Verification items for the finished model (mm, model axes). Give positions to 0.01 mm unless a question says otherwise; leave off trailing zeros. Order: outer loops, then holes, each group sorted by start corner. A loop starts at its lowest first (then second) coordinate and runs counter-clockwise, first axis right, second up. Notation, with made-up numbers: (-24, -26.5) - (18, -26.5) arc R13 ccw to (18, -17.5) - close; hole circle Ø11 at (15.25, -17.75). An arc over 180 degrees is marked (long way). Answer as a JSON object with one key per item and string values. Group by question number.
(1) Thickness scan on line 1 (X direction, y = 3, z = 0.8); line 2 (Y direction, x = -50.5, z = 0.75); line 3 (X direction, y = -9.5, z = 0.15). Record the ranges inside material, lowest first.
(2) Section check A-A (z = 0.65). Count the separate pieces of the cut face and the enclosed holes in it, then the cut area to 3 significant figures.
(3) Depth check by flat-ended pin: pin 1 Ø0.5 at (x, z) = (-232.5, 0.5) entering from -Y; pin 2 Ø0.5 at (x, z) = (232.5, 0.5) entering from +Y; pin 3 Ø0.5 at (y, z) = (21, 0.5) entering from -X. Enter the tip coordinate at first touch or a pass-through.
(4) Section check B-B (y = 28). Record the boundary of the cut face in (x, z).
```python
from build123d import *

# Parameters (mm, degrees)
F1_DEPTH = 1
F3_D     = 5
F5_DEPTH = 25
F7_DEPTH = 25


with BuildPart() as f1:
    # F0 (on Top) → F1 (new body)
    with BuildSketch(Plane.XY):
        Polygon((221, 20), (221, 33.5), (0, 33.5), (-221, 33.5), (-221, 20), (-223, 20), (-223, 22), (-239, 22), (-241, 20), (-241, 0), (-241, -20), (-239, -22), (-223, -22), (-223, -20), (-221, -20), (-221, -33.5), (0, -33.5), (221, -33.5), (221, -20), (223, -20), (223, -22), (239, -22), (241, -20), (241, 0), (241, 20), (239, 22), (223, 22), (223, 20), align=None)
    extrude(amount=F1_DEPTH)

    # F3 (through all)
    with Locations(Plane.XY.offset(1)):
        with Locations((-200, 0), (-100, 0), (0, 0), (100, 0), (200, 0)):
            Hole(F3_D / 2)

    # F4 (on face) → F5 (cut)
    with BuildSketch(Plane.XY.offset(1)):
        with BuildLine():
            Line((-228.9, -13), (-235, -13))
            ThreePointArc((-235, -13), (-238, -16), (-235, -19))
            Line((-235, -19), (-228.9, -19))
            ThreePointArc((-228.9, -19), (-225.9, -16), (-228.9, -13))
        make_face()
        with BuildLine():
            ThreePointArc((-235, 19), (-238, 16), (-235, 13))
            Line((-235, 13), (-228.9, 13))
            ThreePointArc((-228.9, 13), (-225.9, 16), (-228.9, 19))
            Line((-228.9, 19), (-235, 19))
        make_face()
        with BuildLine():
            Line((228.9, 13), (235, 13))
            ThreePointArc((235, 13), (238, 16), (235, 19))
            Line((235, 19), (228.9, 19))
            ThreePointArc((228.9, 19), (225.9, 16), (228.9, 13))
        make_face()
        with BuildLine():
            ThreePointArc((228.9, -13), (225.9, -16), (228.9, -19))
            Line((228.9, -19), (235, -19))
            ThreePointArc((235, -19), (238, -16), (235, -13))
            Line((235, -13), (228.9, -13))
        make_face()
    extrude(amount=-F5_DEPTH, mode=Mode.SUBTRACT)

    # F6 (on face) → F7 (cut)
    with BuildSketch(Plane(origin=(0, 0, 0), x_dir=(1, 0, 0), z_dir=(0, 0, -1))):
        with BuildLine():
            ThreePointArc((120, 12), (116.464466, 10.535534), (115, 7))
            Line((115, 7), (115, -7))
            ThreePointArc((115, -7), (116.464466, -10.535534), (120, -12))
            Line((120, -12), (180, -12))
            ThreePointArc((180, -12), (183.535534, -10.535534), (185, -7))
            Line((185, -7), (185, 7))
            ThreePointArc((185, 7), (183.535534, 10.535534), (180, 12))
            Line((180, 12), (120, 12))
        make_face()
        with BuildLine():
            ThreePointArc((20, 12), (16.464466, 10.535534), (15, 7))
            Line((15, 7), (15, -7))
            ThreePointArc((15, -7), (16.464466, -10.535534), (20, -12))
            Line((20, -12), (80, -12))
            ThreePointArc((80, -12), (83.535534, -10.535534), (85, -7))
            Line((85, -7), (85, 7))
            ThreePointArc((85, 7), (83.535534, 10.535534), (80, 12))
            Line((80, 12), (20, 12))
        make_face()
        with BuildLine():
            ThreePointArc((-15, 7), (-16.464466, 10.535534), (-20, 12))
            Line((-20, 12), (-80, 12))
            ThreePointArc((-80, 12), (-83.535534, 10.535534), (-85, 7))
            Line((-85, 7), (-85, -7))
            ThreePointArc((-85, -7), (-83.535534, -10.535534), (-80, -12))
            Line((-80, -12), (-20, -12))
            ThreePointArc((-20, -12), (-16.464466, -10.535534), (-15, -7))
            Line((-15, -7), (-15, 7))
        make_face()
        with BuildLine():
            ThreePointArc((-115, 7), (-116.464466, 10.535534), (-120, 12))
            Line((-120, 12), (-180, 12))
            ThreePointArc((-180, 12), (-183.535534, 10.535534), (-185, 7))
            Line((-185, 7), (-185, -7))
            ThreePointArc((-185, -7), (-183.535534, -10.535534), (-180, -12))
            Line((-180, -12), (-120, -12))
            ThreePointArc((-120, -12), (-116.464466, -10.535534), (-115, -7))
            Line((-115, -7), (-115, 7))
        make_face()
    extrude(amount=-F7_DEPTH, mode=Mode.SUBTRACT)


solid = f1.part
```
Solutions:
{
 "1": {"line 1": "x = -241 to -185, -115 to -85, -15 to 15, 85 to 115, 185 to 241", "line 2": "y = -33.5 to -12, 12 to 33.5", "line 3": "x = -241 to -184.33, -115.67 to -84.33, -15.67 to 15.67, 84.33 to 115.67, 184.33 to 241"},
 "2": {"separate pieces": "1", "enclosed holes": "13", "area": "24,400 mm2"},
 "3": {"pin 1": "stops at y = -22", "pin 2": "stops at y = 22", "pin 3": "stops at x = -240.25"},
 "4": {"outline": "(-221, 0) - (221, 0) - (221, 1) - (-221, 1) - close"}
}
